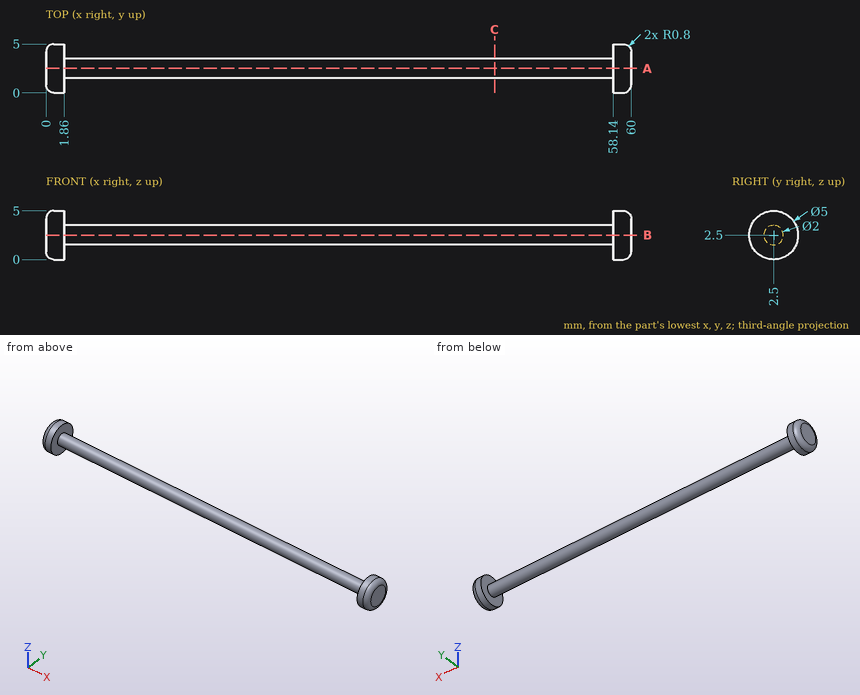
Verification items for this drawing (mm, ordinates from the low corner). Coordinates: 2 decimals unless noted, no trailing zeros. Loops run counter-clockwise (first coordinate to the right, second up) from the corner with the lowest first, then second, coordinate; pieces in that order, holes last. Notation, with made-up numbers: (3.5, -2.5) -> (32.5, -2.5) arc R18 cw to (32.5, 2.5) -> close; hole circle Ø4 at (-14, 30.5). An arc over 180 degrees is marked (long way). Answer in a Markdown table with one row per item. Add a question column.
1. Depth check by flat-ended pin: P1, Ø1.5, axis at x = 20, z = 2, coming from the -Y side; P2, Ø1.5, axis at x = 12, y = 1, coming from the -Z side. Enter the tip coordinate at first touch or a pass-through.
2. Material ranges on probe 1 along X at (y, z) = (1.7, 4); probe 2 along X at (y, z) = (4.6, 3.35); probe 3 along Z at (x, y) = (45.5, 2.55), recorded low to high. Write a range as [from, to].
3. Section check A-A, the plane y = 2.5. Enter the section's corners in (x, z).
4. Section check C-C, the plane x = 46. Enter the section's corners in (y, z), then the cut area to 3 significant figures.
Derived:
| question | item | result |
|---|---|---|
| 1 | P1 | stops at y = 1.5 |
| 1 | P2 | stops at z = 1.84 |
| 2 | probe 1 | x = [0, 1.86], [58.14, 60] |
| 2 | probe 2 | x = [0.23, 1.86], [58.14, 59.77] |
| 2 | probe 3 | z = [1.5, 3.5] |
| 3 | outline | (0, 0.8) arc R0.8 ccw to (0.8, 0) -> (1.86, 0) -> (1.86, 1.5) -> (58.14, 1.5) -> (58.14, 0) -> (59.2, 0) arc R0.8 ccw to (60, 0.8) -> (60, 4.2) arc R0.8 ccw to (59.2, 5) -> (58.14, 5) -> (58.14, 3.5) -> (1.86, 3.5) -> (1.86, 5) -> (0.8, 5) arc R0.8 ccw to (0, 4.2) -> close |
| 4 | outline | circle Ø2 at (2.5, 2.5) |
| 4 | area | 3.14 mm² |
